For this review, take the finished solid that the model builds, in its own axes (mm). Face numbers are marked on the shaded views. A direction names the side the tool comes from. Give positions to 0.01 mm unless a question says otherwise; leave off trailing zeros. Order: outer loops, then holes, each group sorted by start corner. A loop starts at its lowest first (then second) coordinate and runs counter-clockwise, first axis right, second up.
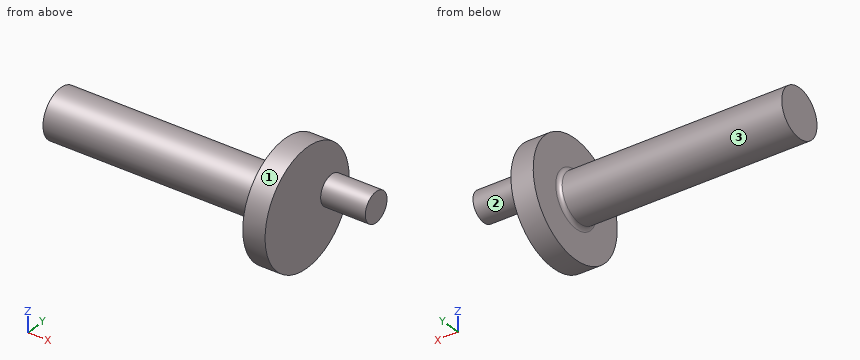
from build123d import *

# Parameters (mm, degrees)
SKETCH1_R           = 15.5
BOSS_EXTRUDE1_DEPTH = 6
SKETCH2_R           = 6.5
BOSS_EXTRUDE2_DEPTH = 60
FILLET1_R           = 1
SKETCH3_R           = 4
BOSS_EXTRUDE3_DEPTH = 12


with BuildPart() as part:
    # Sketch1 → Boss-Extrude1 (new body)
    with BuildSketch(Plane(origin=(0, 0, 0), x_dir=(0, 0, -1), z_dir=(1, 0, 0))):
        Circle(SKETCH1_R)
    extrude(amount=BOSS_EXTRUDE1_DEPTH)

    # Sketch2 → Boss-Extrude2 (add)
    with BuildSketch(Plane.ZY):
        with Locations((0, -0.321626653)):
            Circle(SKETCH2_R)
    extrude(amount=BOSS_EXTRUDE2_DEPTH)

    # Fillet1
    fillet1_edges = [part.edges().sort_by_distance(p)[0] for p in [
        (0, -0.321626653, -6.5),
    ]]
    fillet(fillet1_edges, radius=FILLET1_R)

    # Sketch3 → Boss-Extrude3 (add)
    with BuildSketch(Plane(origin=(6, 0, 0), x_dir=(0, 0, -1), z_dir=(1, 0, 0))):
        with Locations((0, 9)):
            Circle(SKETCH3_R)
    extrude(amount=BOSS_EXTRUDE3_DEPTH)


solid = part.part
1) We need section B-B on y = 8. Give the boundary of the cut face in (x, z), then the cut area to 3 significant figures.
Answer sheet:
outline: (0, -13.28) - (6, -13.28) - (6, -3.87) - (18, -3.87) - (18, 3.87) - (6, 3.87) - (6, 13.28) - (0, 13.28) - close
area: 252 mm2
2) To check wall thickness, follow line 1 (X direction, y = 0, z = 2); line 2 (X direction, y = 7.5, z = 6); line 3 (Y direction, x = -12.5, z = -2). State the ranges of each line that lie inside material, in increasing order.
Answer sheet:
line 1: x = -60 to 6
line 2: x = 0 to 6
line 3: y = -6.51 to 5.86
3) We need section C-C on x = 10.5. Give the boundary of the cut face in (y, z), then the cut area to 3 significant figures.
Answer sheet:
outline: circle Ø8 at (9, 0)
area: 50.3 mm2
4) Clearance check with flat-ended pins moving along their axes: pin 1 (5 mm diameter, centred on y = -8.5, z = -10.5, fed in from -X); pin 2 (5 mm diameter, centred on x = 2, y = 5.5, fed in from +Z); pin 3 (5 mm diameter, centred on x = -38.5, z = -2, fed in from -Y). State where each tip first meets the part, or that it passes through.
Answer sheet:
pin 1: stops at x = 0
pin 2: stops at z = 15.21
pin 3: stops at y = -6.82
5) We need section D-D on y = 11.5. Give the boundary of the cut face in (x, z), then the cut area to 3 significant figures.
Answer sheet:
outline: (0, -10.39) - (6, -10.39) - (6, -3.12) - (18, -3.12) - (18, 3.12) - (6, 3.12) - (6, 10.39) - (0, 10.39) - close
area: 200 mm2
6) We need section A-A on z = 0. Give the boundary of the cut face in (x, y).
Answer sheet:
outline: (-60, -6.82) - (-1, -6.82) arc R1 cw to (0, -7.82) - (0, -15.5) - (6, -15.5) - (6, 5) - (18, 5) - (18, 13) - (6, 13) - (6, 15.5) - (0, 15.5) - (0, 7.18) arc R1 cw to (-1, 6.18) - (-60, 6.18) - close
7) Tool access review of the marked faces 1, 2 and 3: name each direction out of +Z, -Z, +X, -X, +Y, -Y from which nothing blocks a thin tool from reaching the whole face with its end or side.
Answer sheet:
face 1: +X, -X
face 2: +X
face 3: -X
